from build123d import *

# Parameters (mm, degrees)
F0_R     = 8.75
F1_DEPTH = 1
F2_R     = 7.25
F3_DEPTH = 3.6
F4_R     = 6.5
F5_DEPTH = 2.6
F6_R     = 3.625
F7_DEPTH = 2.001


with BuildPart() as f1:
    # F0 (on Top) → F1 (new body)
    with BuildSketch(Plane.XY):
        Circle(F0_R)
    extrude(amount=F1_DEPTH)

    # F2 (on face) → F3 (join)
    with BuildSketch(Plane.XY.offset(1)):
        Circle(F2_R)
    extrude(amount=F3_DEPTH)

    # F4 (on face) → F5 (cut)
    with BuildSketch(Plane.XY.offset(4.6)):
        Circle(F4_R)
    extrude(amount=-F5_DEPTH, mode=Mode.SUBTRACT)

    # F6 (on face) → F7 (cut, through all)
    with BuildSketch(Plane.XY.offset(2)):
        Circle(F6_R)
    extrude(amount=-F7_DEPTH, mode=Mode.SUBTRACT)


solid = f1.part
Work out the finished part from the listing and answer in its coordinate system (mm). A direction names the side the tool comes from. Round coordinates to 2 decimals unless told otherwise and drop trailing zeros. Loops run counter-clockwise (first coordinate to the right, second up) from the corner with the lowest first, then second, coordinate; pieces in that order, holes last. Notation, with made-up numbers: (-20.5, 78) -> (26.5, 78) arc R10 ccw to (26.5, 97) -> close; hole circle Ø4 at (63, -31.5). An arc over 180 degrees is marked (long way). Use one line per item in the form item = value.
(1) A tool of negligible diameter and unlimited length cuts with its end or side. For faces 1 (the cylindrical face through (-5.158, -3.955, 3.318)), 2 (the flat face through (-3, 6, 4.6)), from which of +Z, -Z, +X, -X, +Y, -Y can it reach the whole face along a straight path? Write none if from no direction.
Answer list:
face_1 = +Z
face_2 = +Z, +X, -X, +Y, -Y
(2) Find section D-D on y = 4. Give the vertices of the cut face in (x, z).
Answer list:
outline = (-7.78, 0) -> (7.78, 0) -> (7.78, 1) -> (6.05, 1) -> (6.05, 4.6) -> (5.12, 4.6) -> (5.12, 2) -> (-5.12, 2) -> (-5.12, 4.6) -> (-6.05, 4.6) -> (-6.05, 1) -> (-7.78, 1) -> close
(3) Straight lines are drawn through the part: line 1 (Y direction, x = 0, z = 3.5); line 2 (Z direction, x = -4.5, y = -7). For each, find the intervals that lie inside material, in ascending order.
Answer list:
line_1 = -7.25 to -6.5, 6.5 to 7.25
line_2 = 0 to 1
(4) Find section A-A on x = 0. Give the vertices of the cut face in (y, z) (3 decimals), then the cut area to 3 significant figures.
Answer list:
outline = (-8.75, 0) -> (-3.625, 0) -> (-3.625, 2) -> (-6.5, 2) -> (-6.5, 4.6) -> (-7.25, 4.6) -> (-7.25, 1) -> (-8.75, 1) -> close; (3.625, 0) -> (8.75, 0) -> (8.75, 1) -> (7.25, 1) -> (7.25, 4.6) -> (6.5, 4.6) -> (6.5, 2) -> (3.625, 2) -> close
area = 21.4 mm2
(5) For a pull along X with two mould halves and no side action, classify faces 3 (the flat face through (-3, 7, 1)), 4 (the cylindrical face through (1.7, -3.2, 1)), 5 (the cylindrical face through (-6.944, -5.324, 0.493)) as released by +X, released by -X, zero draft, split by the parting line, or undercut.
Answer list:
face_3 = zero draft
face_4 = undercut
face_5 = split by the parting line
(6) Find section C-C on z = 1.5. Give the vertices of the cut face in (x, y) (3 decimals), then the cut area to 3 significant figures.
Answer list:
outline = circle Ø14.5 at (0, 0); hole circle Ø7.25 at (0, 0)
area = 124 mm2
(7) Flat-ended cylindrical pins translate along their axes: P1, Ø9.5, axis at x = 0, y = 0, coming from the +Z side; P2, Ø2, axis at y = 3.5, z = 4, coming from the +X side. Find the tip coordinate at first contact, or state that the pin passes through.
Answer list:
P1 = 2
P2 = 6.81
